Autodesk Inventor part; units mm, degrees
ref_plane "YZ Plane" through (0, 0, 0) normal (1, 0, 0) x (0, 1, 0)
ref_plane "XZ Plane" through (0, 0, 0) normal (0, 1, 0) x (-1, 0, 0)
ref_plane "XY Plane" through (0, 0, 0) normal (0, 0, 1) x (1, 0, 0)
sketch "Sketch1" plane through (0, 0, 0) normal (0, 1, 0) x (-1, 0, 0)
  circle A0 centre (0, 0) radius 13.25
  circle A1 centre (0, 0) radius 4
  dimension "d0" = 26.5
  dimension "d1" = 8
extrude "Extrusion1" add sketch "Sketch1" along normal blind 8.5
sketch "Sketch2" plane through (0, 0, 0) normal (0, -1, 0) x (1, 0, 0)
  circle A0 centre (18.5, 0) radius 2.4
  circle A1 centre (-18.5, 0) radius 2.4
  circle A2 centre (18.5, 0) radius 5.25
  circle A3 centre (-18.5, 0) radius 5.25
  line L0 (20.7703, -4.7337) -> (5.7297, -11.9471)
  circle A4 centre (0, 0) radius 13.25
  line L1 (20.7703, 4.7337) -> (5.7297, 11.9471)
  line L2 (-5.7297, -11.9471) -> (-20.7703, -4.7337)
  line L3 (-5.7297, 11.9471) -> (-20.7703, 4.7337)
  point P0 (0, 18.5)
  point P1 (0, -18.5)
  dimension "d6" = 4.8
  dimension "d7" = 4.8
  dimension "d8" = 37
  dimension "d9" = 18.5
  dimension "d10" = 10.5
  dimension "d11" = 10.5
extrude "Extrusion2" add sketch "Sketch2" against normal blind 4.5 contours A2 | A2 A4 L1 | L0 A4 A2 | A4 A3 L3 | L2 A3 A4 | A3
properties part number "O_Do_Lan" material "Brass, Soft Yellow, Welded"
Geometry check sheet. Reference: the model listing, model coordinates, mm. A direction names the side the tool comes from. Give positions to 0.01 mm unless a question says otherwise; leave off trailing zeros. Loops run counter-clockwise (first coordinate to the right, second up) from the corner with the lowest first, then second, coordinate; pieces in that order, holes last. Notation, with made-up numbers: (89.25, 56.25) - (127.25, 56.25) arc R10 ccw to (127.25, 68.25) - close; hole circle Ø8 at (59.25, 81). An arc over 180 degrees is marked (long way). Use CSV: the item, a comma, the result in double quotes. Start each with the question number.
Q1. Section check D-D, the plane y = 5.5. Record the cut outline in (x, z).
Q2. Go/stop test with flat-tipped pins: pin 1 Ø3 at (x, y) = (13, 4) entering from -Z; pin 2 Ø10.5 at (x, z) = (0, 0) entering from -Y; pin 3 Ø2 at (x, y) = (-4.5, 1.5) entering from -Z; pin 4 Ø10 at (x, z) = (17, 7.5) entering from +Y. Record where each tip stops, or that it passes through.
Q3. Access from +Z, -Z, +X, -X, +Y, -Y to the whole of each face (thin tool, end or side, straight path). Record for faces 4 (the face through (13.237, 6.079, -0.583)), 5 (the face through (13.355, 2.218, -8.29)).
Q4. Section check B-B, the plane z = 0. Record the cut outline in (x, y), and give its area (3 significant figures).
Q5. Scan lines: probe 1 along Z at (x, y) = (0, 2.5); probe 2 along Y at (x, z) = (-17.5, -5.75); probe 3 along Z at (x, y) = (18.5, 1.55). Record each from-to range of solid material in increasing order. Write a range as from..to.
Q6. Section check C-C, the plane y = 3.25. Record the cut outline in (x, z), and give its area (3 significant figures).
Q7. Section check A-A, the plane x = 0. Record the cut outline in (y, z), and give its area (3 significant figures).
Q8. Release check for a two-part mould opening along Z. For faces 1 (the face through (-17.21, 2.218, 2.024)), 2 (the face through (-13.145, 2.218, -8.391)), 3 (the face through (23.75, 2.22, -0.08)) record: +Z half, -Z half, draft (parallel to the pull), parting line (faces both ways), or undercut.
Findings below:
1,outline,"circle Ø26.5 at (0, 0); hole circle Ø8 at (0, 0)"
2,pin 1,"stops at z = -9.18"
2,pin 2,"stops at y = 0"
2,pin 3,"stops at z = -12.78"
2,pin 4,"stops at y = 4.5"
3,face 4,"+Y"
3,face 5,"-Z, +X, +Y, -Y"
4,outline,"(-23.75, 0) - (-20.9, 0) - (-20.9, 4.5) - (-23.75, 4.5) - close; (-16.1, 0) - (-4, 0) - (-4, 8.5) - (-13.25, 8.5) - (-13.25, 4.5) - (-16.1, 4.5) - close; (4, 0) - (16.1, 0) - (16.1, 4.5) - (13.25, 4.5) - (13.25, 8.5) - (4, 8.5) - close; (20.9, 0) - (23.75, 0) - (23.75, 4.5) - (20.9, 4.5) - close"
4,area,"209 mm^2"
5,probe 1,"z = -13.25..-4, 4..13.25"
5,probe 2,"y = 0..4.5"
5,probe 3,"z = -5.82..-2.4, 2.4..5.82"
6,outline,"(-20.77, -4.73) - (-5.73, -11.95) arc R13.25 ccw to (5.73, -11.95) - (20.77, -4.73) arc R5.25 ccw to (20.77, 4.73) - (5.73, 11.95) arc R13.25 ccw to (-5.73, 11.95) - (-20.77, 4.73) arc R5.25 ccw to start; hole circle Ø4.8 at (-18.5, 0); hole circle Ø8 at (0, 0); hole circle Ø4.8 at (18.5, 0)"
6,area,"750 mm^2"
7,outline,"(0, -13.25) - (8.5, -13.25) - (8.5, -4) - (0, -4) - close; (0, 4) - (8.5, 4) - (8.5, 13.25) - (0, 13.25) - close"
7,area,"157 mm^2"
8,face 1,"undercut"
8,face 2,"-Z half"
8,face 3,"parting line"
